```python
from build123d import *

# Parameters (mm, degrees)
CHAMFER1_SIZE      = 1.5
CUT_EXTRUDE1_DEPTH = 8


with BuildPart() as part:
    # Sketch1 → Revolve1 (revolve)
    with BuildSketch(Plane.XY, mode=Mode.PRIVATE) as revolve1_sk:
        Polygon((0, 0), (4.5, 0), (4.5, 11.5), (6, 11.5), (6, 55), (10.5, 55), (10.5, 70), (0, 70), align=None)
    revolve(revolve1_sk.sketch.rotate(Axis((0, 70, 0), (0, -1, 0)), 180), axis=Axis((0, 70, 0), (0, -1, 0)))

    # Chamfer1
    chamfer1_edges = [part.edges().sort_by_distance(p)[0] for p in [
        (10.5, 70, 0),
        (10.5, 55, 0),
        (6, 11.5, 0),
    ]]
    chamfer(chamfer1_edges, length=CHAMFER1_SIZE - 0.0001)  # a hair under: the kernel refuses the full size

    # Sketch2 → Cut-Extrude1 (cut)
    with BuildSketch(Plane(origin=(0, 70, 0), x_dir=(1, 0, 0), z_dir=(0, 1, 0))):
        Polygon((0, 5.22463141), (-4.524663526, 2.612315705), (-4.524663526, -2.612315705), (0, -5.22463141), (4.524663526, -2.612315705), (4.524663526, 2.612315705), align=None)
    extrude(amount=-CUT_EXTRUDE1_DEPTH, mode=Mode.SUBTRACT)


solid = part.part
```
The model under review builds one solid part; all positions refer to its coordinate system, in mm. A direction names the side the tool comes from. Coordinates: 2 decimals unless noted, no trailing zeros. Order: outer loops, then holes, each group sorted by start corner. A loop starts at its lowest first (then second) coordinate and runs counter-clockwise, first axis right, second up. Notation, with made-up numbers: M -28,-10 L 19,-10 A34 ccw 19,24 Z; hole C -7,18.5 d5. An arc over 180 degrees is marked long. One line per question, with ' | ' between items.
(1) Insertion check: pin 1 (8 mm diameter, centred on x = 2, y = 42.5, fed in from +Z); pin 2 (7 mm diameter, centred on x = -0.5, z = -1.5, fed in from +Y); pin 3 (1 mm diameter, centred on y = 61.5, z = -2, fed in from -X); pin 4 (4 mm diameter, centred on y = 17.5, z = 1, fed in from -X). Each pin has a flat end and moves straight along its axis. Give the tip position at first contact, or say it passes through.
Geometry results:
pin 1: stops at z = 6 | pin 2: stops at y = 70 | pin 3: stops at x = -10.39 | pin 4: stops at x = -6
(2) For probe 1 along Y at (x, z) = (8.25, 3.5); probe 2 along Z at (x, y) = (1.25, 67.5); probe 3 along Y at (x, z) = (2.25, 0.75), list the stretches that pass through material, from the lowest coordinate up. Write a range as from..to.
Geometry results:
probe 1: y = 55..70 | probe 2: z = -10.43..-4.5, 4.5..10.43 | probe 3: y = 0..62
(3) Machinability: for faces 1 (the face through (3.32, 5.83, -3.04)), 2 (the face through (0, 0, 0)), 3 (the face through (-2.231, 66.056, -3.937)), which of the approach directions +Z, -Z, +X, -X, +Y, -Y give a long, thin tool a straight path to every point of the face, cutting with its end or side? Answer none if there is none.
Geometry results:
face 1: -Y | face 2: +Z, -Z, +X, -X, -Y | face 3: +Y
(4) The part is to be moulded in two halves that separate along X. For faces 4 (the face through (2, 55, 6)), 5 (the face through (-2.294, 66.056, 3.9)), 6 (the face through (-10, 62.6, -3.2)), 7 (the face through (-4.525, 66, 0)), say which applies: +X half, -X half, draft (parallel to the pull), parting line (faces both ways), or undercut.
Geometry results:
face 4: draft | face 5: undercut | face 6: parting line | face 7: undercut
(5) Add section B-B, the plane y = 33.5. Write out the cut boundary in (x, z), then the cut area to 3 significant figures.
Geometry results:
outline: C 0,0 d12 | area: 113 mm²
